Work out the finished part from the listing and answer in its coordinate system (mm). A direction names the side the tool comes from. Round coordinates to 2 decimals unless told otherwise and drop trailing zeros. Loops run counter-clockwise (first coordinate to the right, second up) from the corner with the lowest first, then second, coordinate; pieces in that order, holes last.
```python
from build123d import *

# Parameters (mm, degrees)
EXTRUDE_1_DEPTH = 3


with BuildPart() as part:
    # 草图1 → 凸台-拉伸1 (new body)
    with BuildSketch(Plane.XY):
        with BuildLine():
            Line((-4.9, 107.9), (104.9, 107.9))
            ThreePointArc((104.9, 107.9), (107.021320344, 107.021320344), (107.9, 104.9))
            Line((107.9, 104.9), (107.9, -4.9))
            ThreePointArc((107.9, -4.9), (107.021320344, -7.021320344), (104.9, -7.9))
            Line((104.9, -7.9), (-4.9, -7.9))
            ThreePointArc((-4.9, -7.9), (-7.021320344, -7.021320344), (-7.9, -4.9))
            Line((-7.9, -4.9), (-7.9, 104.9))
            ThreePointArc((-7.9, 104.9), (-7.021320344, 107.021320344), (-4.9, 107.9))
        make_face()
        Polygon((100, -2.9), (0, -2.9), (0, 0), (-2.9, 0), (-2.9, 100), (0, 100), (0, 102.9), (100, 102.9), (100, 100), (102.9, 100), (102.9, 0), (100, 0), align=None, mode=Mode.SUBTRACT)
    extrude(amount=EXTRUDE_1_DEPTH)


solid = part.part
```
1. Consider probe 1 along X at (y, z) = (27, 2.1); probe 2 along X at (y, z) = (102.5, 2.8). Determine where each line is inside the solid, lowest interval first.
Answer key:
probe 1: x = -7.9 to -2.9, 102.9 to 107.9
probe 2: x = -7.9 to 0, 100 to 107.9
2. Find section C-C (z = 1.55). Write down the section's boundary in (x, y).
Answer key:
outline: (-7.9, -4.9) arc R3 ccw to (-4.9, -7.9) - (104.9, -7.9) arc R3 ccw to (107.9, -4.9) - (107.9, 104.9) arc R3 ccw to (104.9, 107.9) - (-4.9, 107.9) arc R3 ccw to (-7.9, 104.9) - close; hole (-2.9, 0) - (0, 0) - (0, -2.9) - (100, -2.9) - (100, 0) - (102.9, 0) - (102.9, 100) - (100, 100) - (100, 102.9) - (0, 102.9) - (0, 100) - (-2.9, 100) - close
3. Determine the mould class of faces 1 (the face through (107, 107.04, 1.48)), 2 (the face through (-1, 100, 1)), 3 (the face through (-7.04, 107, 1.48)) for opening direction X: +X half, -X half, draft (parallel to the pull), parting line (faces both ways), or undercut.
Answer key:
face 1: +X half
face 2: undercut
face 3: -X half
4. Which of the six approach directions +Z, -Z, +X, -X, +Y, -Y give full straight-line access (tool end or side, diameter ignored) to faces 4 (the face through (100, 101, 1)), 5 (the face through (51, -7.9, 1))?
Answer key:
face 4: +Z, -Z
face 5: +Z, -Z, +X, -X, -Y
5. Find section A-A (x = 41). Write down the section's boundary in (y, z).
Answer key:
outline: (-7.9, 0) - (-2.9, 0) - (-2.9, 3) - (-7.9, 3) - close; (102.9, 0) - (107.9, 0) - (107.9, 3) - (102.9, 3) - close
